Could you check a few things on this model? Use its own coordinates, in mm. A direction names the side the tool comes from. Give positions to 0.01 mm unless a question says otherwise; leave off trailing zeros. Write each loop counter-clockwise with the first axis right and the second up, starting at its lowest first coordinate (ties: lowest second). Pieces come first, ordered by that corner, then holes. Notation, with made-up numbers: M 67.25,-26.75 L 121.25,-26.75 A18 ccw 121.25,-20.75 Z; hole C 70,-31.75 d10. An arc over 180 degrees is marked long. One line per item, written item: value.
Autodesk Inventor part; units mm, degrees
ref_plane "YZ Plane" through (0, 0, 0) normal (1, 0, 0) x (0, 1, 0)
ref_plane "XZ Plane" through (0, 0, 0) normal (0, 1, 0) x (-1, 0, 0)
ref_plane "XY Plane" through (0, 0, 0) normal (0, 0, 1) x (1, 0, 0)
sketch "Sketch1" plane through (0, 0, 0) normal (0, 0, 1) x (1, 0, 0)
  line L0 (-12.1705, 0) -> (76.7295, 0)
  line L1 (76.7295, 0) -> (76.7295, 9.525)
  line L2 (76.7295, 9.525) -> (51.3295, 9.525)
  line L3 (-12.1705, 0) -> (-12.1705, 9.525)
  line L4 (-12.1705, 9.525) -> (13.2295, 9.525)
  line L5 (13.2295, 9.525) -> (13.2295, 34.925)
  line L6 (51.3295, 9.525) -> (51.3295, 34.925)
  line L7 (13.2295, 34.925) -> (25.9295, 34.925)
  line L8 (25.9295, 34.925) -> (25.9295, 9.525)
  line L9 (25.9295, 9.525) -> (38.6295, 9.525)
  line L10 (38.6295, 9.525) -> (38.6295, 34.925)
  line L11 (38.6295, 34.925) -> (51.3295, 34.925)
  point P0 (0, 0)
  dimension "d0" = 88.9
  dimension "d1" = 9.525
  dimension "d2" = 25.4
  dimension "d3" = 25.4
  dimension "d4" = 25.4
  dimension "d8" = 12.7
  dimension "d9" = 12.7
extrude "Extrusion1" add sketch "Sketch1" against normal blind 50.8
sketch "Sketch2" plane through (51.3295, 9.525, 0) normal (0, 1, 0) x (1, 0, 0)
  line L0 (25.4, 50.8) -> (0, 50.8)
  line L1 (25.4, 0) -> (25.4, 50.8)
  line L2 (-63.5, 0) -> (-63.5, 50.8)
  point P0 (-51.3295, 0)
  point P1 (19.05, 12.7)
  point P2 (19.05, 38.1)
  point P3 (-57.15, 38.1)
  point P4 (-57.15, 12.7)
  dimension "d12" = 6.35
  dimension "d13" = 6.35
  dimension "d14" = 25.4
  dimension "d15" = 12.7
sketch "Sketch3" plane through (51.3295, 9.525, 0) normal (1, 0, 0) x (0, 0, -1)
  line L0 (0, 25.4) -> (50.8, 25.4)
  line L1 (0, 0) -> (0, 25.4)
  point P0 (0, -9.525)
  point P1 (6.35, 12.7)
  point P2 (15.875, 12.7)
  point P3 (25.4, 12.7)
  point P4 (34.925, 12.7)
  point P5 (44.45, 12.7)
  dimension "d23" = 9.525
  dimension "d24" = 9.525
  dimension "d25" = 9.525
  dimension "d26" = 9.525
  dimension "d27" = 12.7
  dimension "d28" = 6.35
hole "Hole1" at (-5.8205, 9.525, -12.7) at (-5.8205, 9.525, -38.1) at (70.3795, 9.525, -38.1) at (70.3795, 9.525, -12.7) direction (0, -1, 0) diameter 6.35 depth 25.4 tip angle 118
hole "Hole2" at (51.3295, 22.225, -6.35) at (51.3295, 22.225, -15.875) at (51.3295, 22.225, -25.4) at (51.3295, 22.225, -34.925) at (51.3295, 22.225, -44.45) direction (-1, 0, 0) diameter 4.7625 depth 25.4 tip angle 118
properties part number "solid_alum_chain_grabber"
1) On a 3-axis mill with a long thin cutter (end or side, diameter ignored), from which of +Z, -Z, +X, -X, +Y, -Y can I reach the whole of each face in a straight line? I mean faces 1 (the face through (44.89, 20.62, -4.59)), 2 (the face through (32, 9.525, -25)), 3 (the face through (51.33, 19, -25)). Say none if no direction works.
Outcome:
face 1: +X
face 2: +Z, -Z, +Y
face 3: +Z, -Z, +X, +Y
2) Please list where these lines run through material, in increasing order: L1, parallel to X at y = 3, z = -38.1; L2, parallel to X at y = 15, z = -24.5; L3, parallel to X at y = 5, z = -41. Write a range as from..to.
Outcome:
L1: x = -12.17..-9, -2.65..67.2, 73.55..76.73
L2: x = 13.23..25.93, 38.63..51.33
L3: x = -12.17..-7.11, -4.53..69.09, 71.67..76.73
3) If we section it at B-B, the plane y = 6: Give the number of separate pieces and of enclosed holes in the cut face, then the cut area to 3 significant figures.
Outcome:
separate pieces: 1
enclosed holes: 4
area: 4,390 mm^2
4) If we section it at A-A, the plane y = 14: Write out the boundary of the cut face in (x, z).
Outcome:
outline: M 13.23,-50.8 L 25.93,-50.8 L 25.93,0 L 13.23,0 Z; M 38.63,-50.8 L 51.33,-50.8 L 51.33,0 L 38.63,0 Z
5) If we section it at C-C, the plane x = 60.5: Write out the boundary of the cut face in (y, z) (3 decimals), then the cut area to 3 significant figures.
Outcome:
outline: M 0,-50.8 L 9.525,-50.8 L 9.525,0 L 0,0 Z
area: 484 mm^2
6) I'm going to push flat-ended pins straight in: pin 1 (2 mm diameter, centred on x = 27.5, y = 9, fed in from +Z); pin 2 (20.5 mm diameter, centred on x = -5, z = -17, fed in from +Y) (3 decimals); pin 3 (5 mm diameter, centred on y = 17.5, z = -16, fed in from +X); pin 4 (7.5 mm diameter, centred on y = 22.225, z = -15.875, fed in from -X). Where does each tip first touch, or does it pass through?
Outcome:
pin 1: stops at z = 0
pin 2: stops at y = 9.525
pin 3: stops at x = 51.33
pin 4: stops at x = 13.23
7) We'd pull the mould along Y, two halves only. Please class faces 4 (the face through (25.93, 19.6, -25)), 5 (the face through (24.747, 22.349, -6.744)), 6 (the face through (45, 34.925, -25)): pulls with the +Y half, pulls with the -Y half, needs draft (parallel to the pull), parting line crosses it, or undercut.
Outcome:
face 4: needs draft
face 5: undercut
face 6: pulls with the +Y half
